Could you check a few things on this model? Use its own coordinates, in mm. A direction names the side the tool comes from. Coordinates: 2 decimals unless noted, no trailing zeros. Loops run counter-clockwise (first coordinate to the right, second up) from the corner with the lowest first, then second, coordinate; pieces in that order, holes last.
from build123d import *

# Parameters (mm, degrees)
SKETCH1_R           = 1.35
SKETCH1_R_2         = 1.524
BOSS_EXTRUDE1_DEPTH = 0.8
SKETCH2_R           = 1.625
SKETCH2_R_2         = 12
CUT_EXTRUDE1_DEPTH  = 51.919642575
BOSS_EXTRUDE2_DEPTH = 1.6
CUT_EXTRUDE2_DEPTH  = 60.521508717


with BuildPart() as part:
    # Sketch1 → Boss-Extrude1 (new, symmetric)
    with BuildSketch(Plane.XY):
        with BuildLine():
            Line((22.5, 25), (22.5, -25))
            ThreePointArc((22.5, -25), (21.621320344, -27.121320344), (19.5, -28))
            Line((19.5, -28), (-39.5, -28))
            ThreePointArc((-39.5, -28), (-41.621320344, -27.121320344), (-42.5, -25))
            Line((-42.5, -25), (-42.5, 25))
            ThreePointArc((-42.5, 25), (-41.621320344, 27.121320344), (-39.5, 28))
            Line((-39.5, 28), (19.5, 28))
            ThreePointArc((19.5, 28), (21.621320344, 27.121320344), (22.5, 25))
        make_face()
        with Locations((-39, 24.5)):
            Circle(SKETCH1_R, mode=Mode.SUBTRACT)
        with Locations((-39, -24.5)):
            Circle(SKETCH1_R_2, mode=Mode.SUBTRACT)
        with Locations((19, -24.5)):
            Circle(SKETCH1_R_2, mode=Mode.SUBTRACT)
        with Locations((19, 24.5)):
            Circle(SKETCH1_R, mode=Mode.SUBTRACT)
    extrude(amount=BOSS_EXTRUDE1_DEPTH, both=True)

    # Sketch2 → Cut-Extrude1 (cut, through all)
    with BuildSketch(Plane.XY.offset(0.8)):
        with Locations((-2.799944405, 16.10995525)):
            Circle(SKETCH2_R)
        with Locations((-22.799944405, 16.10995525)):
            Circle(SKETCH2_R)
        with Locations((-22.799944405, -3.89004475)):
            Circle(SKETCH2_R)
        with Locations((-2.799944405, -3.89004475)):
            Circle(SKETCH2_R)
        with Locations((-12.799944405, 6.10995525)):
            Circle(SKETCH2_R_2)
    extrude(amount=-CUT_EXTRUDE1_DEPTH, mode=Mode.SUBTRACT)

    # Sketch4 → Boss-Extrude2 (add)
    with BuildSketch(Plane.XY.offset(0.8)):
        with BuildLine():
            Line((-49.5, 28), (-39.5, 28))
            ThreePointArc((-39.5, 28), (-41.621320344, 27.121320344), (-42.5, 25))
            Line((-42.5, 25), (-42.5, -25))
            ThreePointArc((-42.5, -25), (-41.621320344, -27.121320344), (-39.5, -28))
            Line((-39.5, -28), (-49.5, -28))
            ThreePointArc((-49.5, -28), (-51.621320344, -27.121320344), (-52.5, -25))
            Line((-52.5, -25), (-52.5, 25))
            ThreePointArc((-52.5, 25), (-51.621320344, 27.121320344), (-49.5, 28))
        make_face()
    extrude(amount=-BOSS_EXTRUDE2_DEPTH)

    # Sketch5 → Cut-Extrude2 (cut, through all)
    with BuildSketch(Plane.XY.offset(0.8)):
        with BuildLine():
            Line((-27.2, -18.8), (-29.6, -18.8))
            Line((-29.6, -18.8), (-29.6, -15.8))
            ThreePointArc((-29.6, -15.8), (-30.3, -15.1), (-31, -15.8))
            Line((-31, -15.8), (-31, -18.14))
            Line((-31, -18.14), (-32.1, -18.14))
            ThreePointArc((-32.1, -18.14), (-32.276776695, -18.213223305), (-32.35, -18.39))
            Line((-32.35, -18.39), (-32.35, -18.8))
            Line((-32.35, -18.8), (-33.5, -18.8))
            ThreePointArc((-33.5, -18.8), (-33.676776695, -18.873223305), (-33.75, -19.05))
            Line((-33.75, -19.05), (-33.75, -28))
            Line((-33.75, -28), (-23.05, -28))
            Line((-23.05, -28), (-23.05, -19.05))
            ThreePointArc((-23.05, -19.05), (-23.123223305, -18.873223305), (-23.3, -18.8))
            Line((-23.3, -18.8), (-24.45, -18.8))
            Line((-24.45, -18.8), (-24.45, -18.39))
            ThreePointArc((-24.45, -18.39), (-24.523223305, -18.213223305), (-24.7, -18.14))
            Line((-24.7, -18.14), (-25.8, -18.14))
            Line((-25.8, -18.14), (-25.8, -15.8))
            ThreePointArc((-25.8, -15.8), (-26.5, -15.1), (-27.2, -15.8))
            Line((-27.2, -15.8), (-27.2, -18.8))
        make_face()
        with BuildLine():
            Line((-14.2, -18.8), (-16.6, -18.8))
            Line((-16.6, -18.8), (-16.6, -15.8))
            ThreePointArc((-16.6, -15.8), (-17.3, -15.1), (-18, -15.8))
            Line((-18, -15.8), (-18, -18.14))
            Line((-18, -18.14), (-19.1, -18.14))
            ThreePointArc((-19.1, -18.14), (-19.276776695, -18.213223305), (-19.35, -18.39))
            Line((-19.35, -18.39), (-19.35, -18.8))
            Line((-19.35, -18.8), (-20.5, -18.8))
            ThreePointArc((-20.5, -18.8), (-20.676776695, -18.873223305), (-20.75, -19.05))
            Line((-20.75, -19.05), (-20.75, -28))
            Line((-20.75, -28), (-10.05, -28))
            Line((-10.05, -28), (-10.05, -19.05))
            ThreePointArc((-10.05, -19.05), (-10.123223305, -18.873223305), (-10.3, -18.8))
            Line((-10.3, -18.8), (-11.45, -18.8))
            Line((-11.45, -18.8), (-11.45, -18.39))
            ThreePointArc((-11.45, -18.39), (-11.523223305, -18.213223305), (-11.7, -18.14))
            Line((-11.7, -18.14), (-12.8, -18.14))
            Line((-12.8, -18.14), (-12.8, -15.8))
            ThreePointArc((-12.8, -15.8), (-13.5, -15.1), (-14.2, -15.8))
            Line((-14.2, -15.8), (-14.2, -18.8))
        make_face()
        with BuildLine():
            Line((-2.3825, -9.525), (-2.3825, -13.625))
            Line((-2.3825, -13.625), (-4.7475, -13.625))
            Line((-4.7475, -13.625), (-4.7475, -11.525))
            ThreePointArc((-4.7475, -11.525), (-5.2475, -11.025), (-5.7475, -11.525))
            Line((-5.7475, -11.525), (-5.7475, -13.625))
            Line((-5.7475, -13.625), (-7.4825, -13.625))
            ThreePointArc((-7.4825, -13.625), (-7.659276695, -13.698223305), (-7.7325, -13.875))
            Line((-7.7325, -13.875), (-7.7325, -28))
            Line((-7.7325, -28), (-7.426776695, -28))
            Line((-7.426776695, -28), (8.235, -28))
            Line((8.235, -28), (8.235, -13.625613252))
            ThreePointArc((8.235, -13.625613252), (8.226255371, -13.62515336), (8.2175, -13.625))
            Line((8.2175, -13.625), (6.4825, -13.625))
            Line((6.4825, -13.625), (6.4825, -11.525))
            ThreePointArc((6.4825, -11.525), (5.9825, -11.025), (5.4825, -11.525))
            Line((5.4825, -11.525), (5.4825, -13.625))
            Line((5.4825, -13.625), (3.1175, -13.625))
            Line((3.1175, -13.625), (3.1175, -9.525))
            ThreePointArc((3.1175, -9.525), (2.6175, -9.025), (2.1175, -9.525))
            Line((2.1175, -9.525), (2.1175, -13.625))
            Line((2.1175, -13.625), (-1.3825, -13.625))
            Line((-1.3825, -13.625), (-1.3825, -9.525))
            ThreePointArc((-1.3825, -9.525), (-1.8825, -9.025), (-2.3825, -9.525))
        make_face()
    extrude(amount=-CUT_EXTRUDE2_DEPTH, mode=Mode.SUBTRACT)


solid = part.part
(1) Which directions (+Z, -Z, +X, -X, +Y, -Y) give clear straight access to the entire face, cutting with the end or side of a thin tool? Please do faces 4 (the face through (-28, -18.8, 0)), 5 (the face through (-3.152, 14.524, 0.011)).
Answers:
face 4: +Z, -Z, -Y
face 5: +Z, -Z
(2) Imagine slicing it at C-C, the plane z = -0.1. State how many separate pieces and enclosed holes the cut face has, and give its area (3 significant figures).
Answers:
separate pieces: 1
enclosed holes: 9
area: 3,220 mm2
(3) Imagine slicing it at B-B, the plane x = -15.5. Write out the boundary of the cut face in (y, z).
Answers:
outline: (-18.8, -0.8) - (-5.58, -0.8) - (-5.58, 0.8) - (-18.8, 0.8) - close; (17.8, -0.8) - (28, -0.8) - (28, 0.8) - (17.8, 0.8) - close
(4) I need wall thicknesses on probe 1 along Y at (x, z) = (19, -0.15); probe 2 along X at (y, z) = (5.5, 0.5); probe 3 along X at (y, z) = (-4, -0.25). Which ranges of each line are inside material? Lowest first, please.
Answers:
probe 1: y = -28 to -26.02, -22.98 to 23.15, 25.85 to 28
probe 2: x = -52.5 to -24.78, -0.82 to 22.5
probe 3: x = -52.5 to -24.42, -21.18 to -19.26, -6.34 to -4.42, -1.18 to 22.5
(5) Imagine slicing it at A-A, the plane y = 4. Write out the boundary of the cut face in (x, z), and give its area (3 significant figures).
Answers:
outline: (-52.5, -0.8) - (-24.61, -0.8) - (-24.61, 0.8) - (-52.5, 0.8) - close; (-0.99, -0.8) - (22.5, -0.8) - (22.5, 0.8) - (-0.99, 0.8) - close
area: 82.2 mm2
(6) For pin 1 (0.6 mm diameter, centred on x = -12.5, z = 0, fed in from -Y), with a flat end and sliding along its axis, tell me the tip position at first contact or that it passes through.
Answers:
pin 1: stops at y = -18.14
(7) We'd pull the mould along X, two halves only. Please class faces 1 (the face through (-51.6, -27.14, 0.01)), 2 (the face through (-15, 28, 0)), 3 (the face through (-18, -17, 0)): +X half, -X half, draft (parallel to the pull), parting line (faces both ways), or undercut.
Answers:
face 1: -X half
face 2: draft
face 3: undercut
